Could you check a few things on this model? Use its own coordinates, in mm. Face numbers are marked on the shaded views. A direction names the side the tool comes from. Coordinates: 2 decimals unless noted, no trailing zeros. Loops run counter-clockwise (first coordinate to the right, second up) from the corner with the lowest first, then second, coordinate; pieces in that order, holes last.
1) Imagine slicing it at A-A on x = 0. Please give me the cut outline in (y, z).
2) Imagine slicing it at B-B on y = -1.5. Please give me the cut outline in (x, z).
3) Will these pins go through, and if not, where does the flat tip stop? P1, Ø1.5, axis at x = 19, z = 0.5, coming from the -Y side; P2, Ø0.9, axis at y = -23.5, z = 0.5, coming from the -X side; P3, Ø1.5, axis at y = 23.5, z = -0.5, coming from the +X side.
4) Thinking about a two-plate mould opening in X: for the marked faces 1, 2 and 3, which applies, released by +X, released by -X, zero draft, split by the parting line, or undercut?
5) For the marked faces 4, 5, 6, 7 and 8, which set-ups out of +Z, -Z, +X, -X, +Y, -Y let a thin tool reach every point of the face, with its end or its side?
6) If I drill on line 1 along Y through (x, z) = (0, -0.75); line 2 along Y through (x, z) = (17, -0.25); line 3 along X through (y, z) = (1.5, 1.35), over which ranges is the centre line in solid material (lowest first)?
```python
from build123d import *

# Parameters (mm, degrees)
BOSS_EXTRUDE1_DEPTH = 1.5
BOSS_EXTRUDE2_DEPTH = 1.5
CIRPATTERN1_COUNT   = 18


with BuildPart() as part:
    # Sketch1 → Boss-Extrude1 (new, symmetric)
    with BuildSketch(Plane.XY):
        with BuildLine():
            ThreePointArc((1.5, 22.449944321), (0, 22.5), (-1.5, 22.449944321))
            ThreePointArc((-1.5, 22.449944321), (-15.370426149, -16.431676725), (22.5, 0))
            ThreePointArc((22.5, 0), (16.431676725, 15.370426149), (1.5, 22.449944321))
        make_face()
        with BuildLine():
            ThreePointArc((7.5, 0), (-4.541475531, -5.968668193), (-2, 7.228416147))
            Line((-2, 7.228416147), (-2, 19.228416147))
            Line((-2, 19.228416147), (2, 19.228416147))
            Line((2, 19.228416147), (2, 7.228416147))
            ThreePointArc((2, 7.228416147), (5.968668193, 4.541475531), (7.5, 0))
        make_face(mode=Mode.SUBTRACT)
    extrude(amount=BOSS_EXTRUDE1_DEPTH, both=True)

    # Sketch1_3 → Boss-Extrude2 (add, symmetric)
    with BuildSketch(Plane.XY):
        with BuildLine():
            Line((-1.5, 25.449944321), (-1.5, 22.449944321))
            ThreePointArc((-1.5, 22.449944321), (0, 22.5), (1.5, 22.449944321))
            Line((1.5, 22.449944321), (1.5, 25.449944321))
            Line((1.5, 25.449944321), (-1.5, 25.449944321))
        make_face()
    boss_extrude2 = extrude(amount=BOSS_EXTRUDE2_DEPTH, both=True)

    # CirPattern1: Boss-Extrude2 ×18 about axis
    cirpattern1_axis = Axis((0, 0, 0), (0, 0, 1))
    for i in range(1, CIRPATTERN1_COUNT):
        add(boss_extrude2.rotate(cirpattern1_axis, i * 360 / CIRPATTERN1_COUNT))


solid = part.part
```
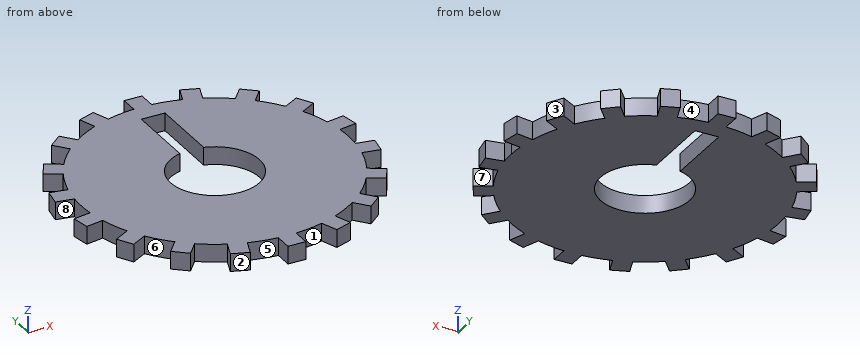
Filled in:
1. outline: (-25.45, -1.5) - (-7.5, -1.5) - (-7.5, 1.5) - (-25.45, 1.5) - close; (19.23, -1.5) - (25.45, -1.5) - (25.45, 1.5) - (19.23, 1.5) - close
2. outline: (-22.45, -1.5) - (-7.35, -1.5) - (-7.35, 1.5) - (-22.45, 1.5) - close; (7.35, -1.5) - (22.45, -1.5) - (22.45, 1.5) - (7.35, 1.5) - close
3. P1: stops at y = -13.16
3. P2: stops at x = -10.11
3. P3: stops at x = 10.11
4. face 1: undercut
4. face 2: released by -X
4. face 3: released by +X
5. face 4: +Z, -Z, +Y
5. face 5: +Z, -Z, -Y
5. face 6: +Z, -Z
5. face 7: +Z, -Z, +X
5. face 8: +Z, -Z, -X
6. line 1: y = -25.45 to -7.5, 19.23 to 25.45
6. line 2: y = -18.96 to -17.93, -14.74 to 14.74, 17.93 to 18.96
6. line 3: x = -22.45 to -7.35, 7.35 to 22.45
